Work out the finished part from the listing and answer in its coordinate system (mm). Coordinates: 2 decimals unless noted, no trailing zeros. Order: outer loops, then holes, each group sorted by start corner. A loop starts at its lowest first (then second) coordinate and runs counter-clockwise, first axis right, second up.
1. Find the intervals of material crossed by probe 1 along X at (y, z) = (37, 2.5); probe 2 along Y at (x, z) = (-14.5, 2.2); probe 3 along Z at (x, y) = (-18, 44), in increasing order.
2. The part is cut by section A-A, the plane x = 18. Give the vertices of the cut face in (y, z), then the cut area to 3 significant figures.
3. Flat-ended cylindrical pins translate along their axes: pin 1 Ø4 at (x, y) = (59.96, 32.56) entering from +Z; pin 2 Ø3 at (x, y) = (38.03, 37.16) entering from -Z; pin 3 Ø2 at (y, z) = (-10.5, 1.5) entering from +X; pin 4 Ø0.5 at (x, y) = (14, 39) entering from -Z. Find the tip coordinate at first contact, or state that the pin passes through.
4. The part is cut by section C-C, the plane x = 4.5. Give the vertices of the cut face in (y, z), then the cut area to 3 significant figures.
5. The part is cut by section B-B, the plane y = 0. Give the vertices of the cut face in (x, z), then the cut area to 3 significant figures.
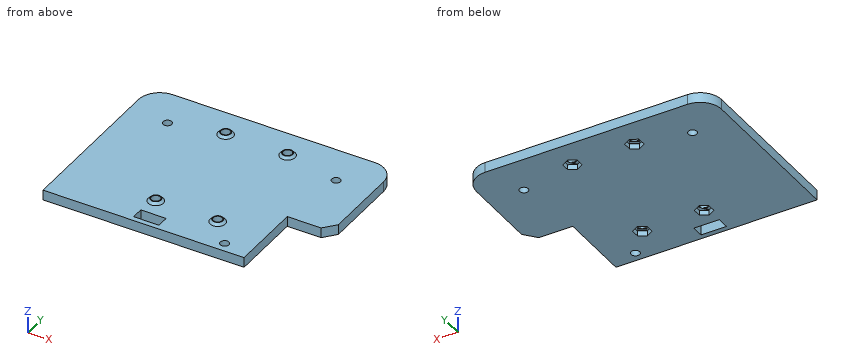
```python
from build123d import *
from OCP.BRepFilletAPI import BRepFilletAPI_MakeChamfer

# Parameters (mm, degrees)
CROQUIS1_R              = 1.7
CROQUIS1_W              = 10.058265445
CROQUIS1_H              = 4.759112173
SALIENTE_EXTRUIR1_DEPTH = 4
CROQUIS2_R              = 3
CROQUIS2_R_2            = 1.75
SALIENTE_EXTRUIR2_DEPTH = 1
CHAFL_N1_SIZE           = 1
CHAFL_N1_SIZE_2         = 0.932515086
CORTAR_EXTRUIR1_START   = -6
CROQUIS3_R              = 1.75
CORTAR_EXTRUIR1_DEPTH   = 6
CORTAR_EXTRUIR2_DEPTH   = 2
CORTAR_EXTRUIR3_DEPTH   = 0.2
CORTAR_EXTRUIR4_DEPTH   = 0.2


with BuildPart() as part:
    # Croquis1 → Saliente-Extruir1 (new body)
    with BuildSketch(Plane.XY):
        with BuildLine():
            Line((46.761077919, -23.458131852), (56.832754836, -23.458131852))
            Line((56.832754836, -23.458131852), (56.832754836, 5.314653818))
            Line((56.832754836, 5.314653818), (70.245248308, 5.314653818))
            Line((70.245248308, 5.314653818), (74.283027827, 9.974351882))
            Line((74.283027827, 9.974351882), (74.283027827, 40))
            ThreePointArc((74.283027827, 40), (71.793435467, 46.01040764), (65.783027827, 48.5))
            Line((65.783027827, 48.5), (-14.216972173, 48.5))
            ThreePointArc((-14.216972173, 48.5), (-20.227379813, 46.01040764), (-22.716972173, 40))
            Line((-22.716972173, 40), (-22.716972173, -23.458131852))
            Line((-22.716972173, -23.458131852), (46.761077919, -23.458131852))
        make_face()
        with Locations((46.761077919, -19.458131852)):
            Circle(CROQUIS1_R, mode=Mode.SUBTRACT)
        with Locations((-7.00634082, 32.938725209)):
            Circle(CROQUIS1_R, mode=Mode.SUBTRACT)
        with Locations((59.964675143, 32.558212342)):
            Circle(CROQUIS1_R, mode=Mode.SUBTRACT)
        with Locations((16.969290087, -19.074136319)):
            Rectangle(CROQUIS1_W, CROQUIS1_H, mode=Mode.SUBTRACT)
    extrude(amount=SALIENTE_EXTRUIR1_DEPTH)

    # Croquis2 → Saliente-Extruir2 (add)
    # profile 1 of 4: a face of its own
    with BuildSketch(Plane.XY.offset(4)):
        with Locations((13.527577906, 37.15608476)):
            Circle(CROQUIS2_R)
        with Locations((13.527577906, 37.15608476)):
            Circle(CROQUIS2_R_2, mode=Mode.SUBTRACT)
    # profile 2 of 4: a face of its own
    with BuildSketch(Plane.XY.offset(4)):
        with Locations((38.027577906, 37.15608476)):
            Circle(CROQUIS2_R)
        with Locations((38.027577906, 37.15608476)):
            Circle(CROQUIS2_R_2, mode=Mode.SUBTRACT)
    # profile 3 of 4: a face of its own
    with BuildSketch(Plane.XY.offset(4)):
        with Locations((38.027577906, -9.34391524)):
            Circle(CROQUIS2_R)
        with Locations((38.027577906, -9.34391524)):
            Circle(CROQUIS2_R_2, mode=Mode.SUBTRACT)
    # profile 4 of 4: a face of its own
    with BuildSketch(Plane.XY.offset(4)):
        with Locations((13.527577906, -9.34391524)):
            Circle(CROQUIS2_R)
        with Locations((13.527577906, -9.34391524)):
            Circle(CROQUIS2_R_2, mode=Mode.SUBTRACT)
    extrude(amount=SALIENTE_EXTRUIR2_DEPTH)

    # Chaflán1
    chafl_n1_edges_1 = [part.edges().sort_by_distance(p)[0] for p in [
        (10.527577906, 37.15608476, 5),
    ]]
    chafl_n1_side_1 = [part.faces().sort_by_distance(p)[0] for p in [
        (10.527577906, 37.15608476, 4.981349698),
    ]]
    chafl_n1_edges_2 = [part.edges().sort_by_distance(p)[0] for p in [
        (35.027577906, 37.15608476, 5),
    ]]
    chafl_n1_side_2 = [part.faces().sort_by_distance(p)[0] for p in [
        (35.027577906, 37.15608476, 4.981349698),
    ]]
    chafl_n1_edges_3 = [part.edges().sort_by_distance(p)[0] for p in [
        (35.027577906, -9.34391524, 5),
    ]]
    chafl_n1_side_3 = [part.faces().sort_by_distance(p)[0] for p in [
        (35.027577906, -9.34391524, 4.981349698),
    ]]
    chafl_n1_edges_4 = [part.edges().sort_by_distance(p)[0] for p in [
        (10.527577906, -9.34391524, 5),
    ]]
    chafl_n1_side_4 = [part.faces().sort_by_distance(p)[0] for p in [
        (10.527577906, -9.34391524, 4.981349698),
    ]]
    chafl_n1 = BRepFilletAPI_MakeChamfer(part.part.solid().wrapped)
    for e in chafl_n1_edges_1:
        chafl_n1.Add(CHAFL_N1_SIZE - 0.0001, CHAFL_N1_SIZE_2 - 0.0001, e.wrapped, chafl_n1_side_1[0].wrapped)
    for e in chafl_n1_edges_2:
        chafl_n1.Add(CHAFL_N1_SIZE - 0.0001, CHAFL_N1_SIZE_2 - 0.0001, e.wrapped, chafl_n1_side_2[0].wrapped)
    for e in chafl_n1_edges_3:
        chafl_n1.Add(CHAFL_N1_SIZE - 0.0001, CHAFL_N1_SIZE_2 - 0.0001, e.wrapped, chafl_n1_side_3[0].wrapped)
    for e in chafl_n1_edges_4:
        chafl_n1.Add(CHAFL_N1_SIZE - 0.0001, CHAFL_N1_SIZE_2 - 0.0001, e.wrapped, chafl_n1_side_4[0].wrapped)
    add(Compound.cast(chafl_n1.Shape()), mode=Mode.REPLACE)  # a hair under: the kernel refuses the full size

    # Croquis3 → Cortar-Extruir1 (cut)
    with BuildSketch(Plane.XY.offset(4).offset(CORTAR_EXTRUIR1_START)):
        with Locations((13.527577906, -9.34391524)):
            Circle(CROQUIS3_R)
        with Locations((38.027577906, -9.34391524)):
            Circle(CROQUIS3_R)
        with Locations((38.027577906, 37.15608476)):
            Circle(CROQUIS3_R)
        with Locations((13.527577906, 37.15608476)):
            Circle(CROQUIS3_R)
    extrude(amount=CORTAR_EXTRUIR1_DEPTH, mode=Mode.SUBTRACT)

    # Croquis5 → Cortar-Extruir2 (cut)
    with BuildSketch(Plane(origin=(0, 0, 0), x_dir=(-1, 0, 0), z_dir=(0, 0, -1))):
        Polygon((-13.528313647, -12.655938197), (-10.653313647, -10.996056173), (-10.653313647, -7.676292125), (-13.528313647, -6.016410101), (-16.403313647, -7.676292125), (-16.403313647, -10.996056173), align=None)
        Polygon((-40.868755289, -7.676292125), (-37.993755289, -6.016410101), (-35.118755289, -7.676292125), (-35.118755289, -10.996056173), (-37.993755289, -12.655938197), (-40.868755289, -10.996056173), align=None)
        Polygon((-40.868755289, 38.845431555), (-40.868755289, 35.525667507), (-37.993755289, 33.865785483), (-35.118755289, 35.525667507), (-35.118755289, 38.845431555), (-37.993755289, 40.505313579), align=None)
        Polygon((-16.403313647, 35.525667507), (-16.403313647, 38.845431555), (-13.528313647, 40.505313579), (-10.653313647, 38.845431555), (-10.653313647, 35.525667507), (-13.528313647, 33.865785483), align=None)
    extrude(amount=-CORTAR_EXTRUIR2_DEPTH, mode=Mode.SUBTRACT)

    # Croquis6 → Cortar-Extruir3 (cut)
    with BuildSketch(Plane(origin=(0, 0, 2), x_dir=(-1, 0, 0), z_dir=(0, 0, -1))):
        with BuildLine():
            Line((-14.680313514, -10.660615896), (-13.528313647, -12.655938197))
            Line((-13.528313647, -12.655938197), (-10.653313647, -10.996056173))
            Line((-10.653313647, -10.996056173), (-11.814996998, -8.983961587))
            ThreePointArc((-11.814996998, -8.983961587), (-11.786957817, -9.162968548), (-11.777577906, -9.34391524))
            ThreePointArc((-11.777577906, -9.34391524), (-12.804662736, -10.937619622), (-14.680313514, -10.660615896))
        make_face()
        with BuildLine():
            Line((-16.403313647, -7.676292125), (-15.244241928, -9.683863233))
            ThreePointArc((-15.244241928, -9.683863233), (-14.393721726, -7.823292051), (-12.359558444, -8.040753494))
            Line((-12.359558444, -8.040753494), (-13.528313647, -6.016410101))
            Line((-13.528313647, -6.016410101), (-16.403313647, -7.676292125))
        make_face()
        Polygon((-38.026842165, 33.828579621), (-40.901842165, 38.808225692), (-38.026842165, 40.468107716), (-35.151842165, 35.488461645), align=None)
        Polygon((-13.528313647, 40.468107716), (-10.653313647, 38.808225692), (-13.528313647, 33.828579621), (-16.403313647, 35.488461645), align=None)
        Polygon((-38.026842165, -12.655938197), (-40.901842165, -10.996056173), (-38.026842165, -6.016410101), (-35.151842165, -7.676292125), align=None)
    extrude(amount=-CORTAR_EXTRUIR3_DEPTH, mode=Mode.SUBTRACT)

    # Croquis7 → Cortar-Extruir4 (cut)
    with BuildSketch(Plane(origin=(0, 0, 2.2), x_dir=(-1, 0, 0), z_dir=(0, 0, -1))):
        with BuildLine():
            ThreePointArc((-15.244241928, -9.683863233), (-15.11916685, -8.616354498), (-14.393721726, -7.823292051))
            Line((-14.393721726, -7.823292051), (-15.842124921, -8.648299511))
            Line((-15.842124921, -8.648299511), (-15.244241928, -9.683863233))
        make_face()
        with BuildLine():
            Line((-12.962262832, -6.996838873), (-14.393721726, -7.823292051))
            ThreePointArc((-14.393721726, -7.823292051), (-13.341554801, -7.603830356), (-12.359558444, -8.040753494))
            Line((-12.359558444, -8.040753494), (-12.962262832, -6.996838873))
        make_face()
        with BuildLine():
            ThreePointArc((-11.814996998, -8.983961587), (-11.927608639, -10.052856947), (-12.643751504, -10.854329386))
            Line((-12.643751504, -10.854329386), (-11.21229261, -10.027876208))
            Line((-11.21229261, -10.027876208), (-11.814996998, -8.983961587))
        make_face()
        with BuildLine():
            Line((-14.082430521, -11.696179618), (-12.643751504, -10.854329386))
            ThreePointArc((-12.643751504, -10.854329386), (-13.693286293, -11.086052069), (-14.680313514, -10.660615896))
            Line((-14.680313514, -10.660615896), (-14.082430521, -11.696179618))
        make_face()
        with BuildLine():
            ThreePointArc((-39.195597368, -8.040753494), (-38.213601012, -7.603830356), (-37.161434087, -7.823292051))
            Line((-37.161434087, -7.823292051), (-38.592892981, -6.996838873))
            Line((-38.592892981, -6.996838873), (-39.195597368, -8.040753494))
        make_face()
        with BuildLine():
            Line((-36.310913885, -9.683863233), (-35.713030891, -8.648299511))
            Line((-35.713030891, -8.648299511), (-37.161434087, -7.823292051))
            ThreePointArc((-37.161434087, -7.823292051), (-36.435988962, -8.616354498), (-36.310913885, -9.683863233))
        make_face()
        with BuildLine():
            Line((-37.472725291, -11.696179618), (-36.874842298, -10.660615896))
            ThreePointArc((-36.874842298, -10.660615896), (-37.86186952, -11.086052069), (-38.911404308, -10.854329386))
            Line((-38.911404308, -10.854329386), (-37.472725291, -11.696179618))
        make_face()
        with BuildLine():
            Line((-40.342863202, -10.027876208), (-38.911404308, -10.854329386))
            ThreePointArc((-38.911404308, -10.854329386), (-39.627547173, -10.052856947), (-39.740158814, -8.983961587))
            Line((-39.740158814, -8.983961587), (-40.342863202, -10.027876208))
        make_face()
        with BuildLine():
            ThreePointArc((-39.740158814, 36.796131106), (-39.627547173, 37.865026467), (-38.911404308, 38.666498906))
            Line((-38.911404308, 38.666498906), (-40.342863202, 37.840045728))
            Line((-40.342863202, 37.840045728), (-39.740158814, 36.796131106))
        make_face()
        with BuildLine():
            ThreePointArc((-38.911404308, 38.666498906), (-37.86186952, 38.898221589), (-36.874842298, 38.472785416))
            Line((-36.874842298, 38.472785416), (-37.472725291, 39.508349137))
            Line((-37.472725291, 39.508349137), (-38.911404308, 38.666498906))
        make_face()
        with BuildLine():
            ThreePointArc((-36.310913885, 37.496032752), (-36.435988962, 36.428524018), (-37.161434087, 35.635461571))
            Line((-37.161434087, 35.635461571), (-35.713030891, 36.460469031))
            Line((-35.713030891, 36.460469031), (-36.310913885, 37.496032752))
        make_face()
        with BuildLine():
            ThreePointArc((-37.161434087, 35.635461571), (-38.213601012, 35.415999876), (-39.195597368, 35.852923014))
            Line((-39.195597368, 35.852923014), (-38.592892981, 34.809008393))
            Line((-38.592892981, 34.809008393), (-37.161434087, 35.635461571))
        make_face()
        with BuildLine():
            Line((-11.814996998, 36.796131106), (-11.21229261, 37.840045728))
            Line((-11.21229261, 37.840045728), (-12.643751504, 38.666498906))
            ThreePointArc((-12.643751504, 38.666498906), (-11.927608639, 37.865026467), (-11.814996998, 36.796131106))
        make_face()
        with BuildLine():
            ThreePointArc((-14.680313514, 38.472785416), (-13.693286293, 38.898221589), (-12.643751504, 38.666498906))
            Line((-12.643751504, 38.666498906), (-14.082430521, 39.508349137))
            Line((-14.082430521, 39.508349137), (-14.680313514, 38.472785416))
        make_face()
        with BuildLine():
            Line((-15.842124921, 36.460469031), (-14.393721726, 35.635461571))
            ThreePointArc((-14.393721726, 35.635461571), (-15.11916685, 36.428524018), (-15.244241928, 37.496032752))
            Line((-15.244241928, 37.496032752), (-15.842124921, 36.460469031))
        make_face()
        with BuildLine():
            Line((-12.962262832, 34.809008393), (-12.359558444, 35.852923014))
            ThreePointArc((-12.359558444, 35.852923014), (-13.341554801, 35.415999876), (-14.393721726, 35.635461571))
            Line((-14.393721726, 35.635461571), (-12.962262832, 34.809008393))
        make_face()
    extrude(amount=-CORTAR_EXTRUIR4_DEPTH, mode=Mode.SUBTRACT)


solid = part.part
```
Geometry says:
1. probe 1: x = -22.72 to 11.78, 15.27 to 36.28, 39.77 to 74.28
1. probe 2: y = -23.46 to 48.5
1. probe 3: z = 0 to 4
2. outline: (-23.46, 0) - (-21.45, 0) - (-21.45, 4) - (-23.46, 4) - close; (-16.69, 0) - (48.5, 0) - (48.5, 4) - (-16.69, 4) - close
2. area: 269 mm2
3. pin 1: stops at z = 4
3. pin 2: passes through
3. pin 3: stops at x = 56.83
3. pin 4: stops at z = 2.4
4. outline: (-23.46, 0) - (48.5, 0) - (48.5, 4) - (-23.46, 4) - close
4. area: 288 mm2
5. outline: (-22.72, 0) - (56.83, 0) - (56.83, 4) - (-22.72, 4) - close
5. area: 318 mm2
